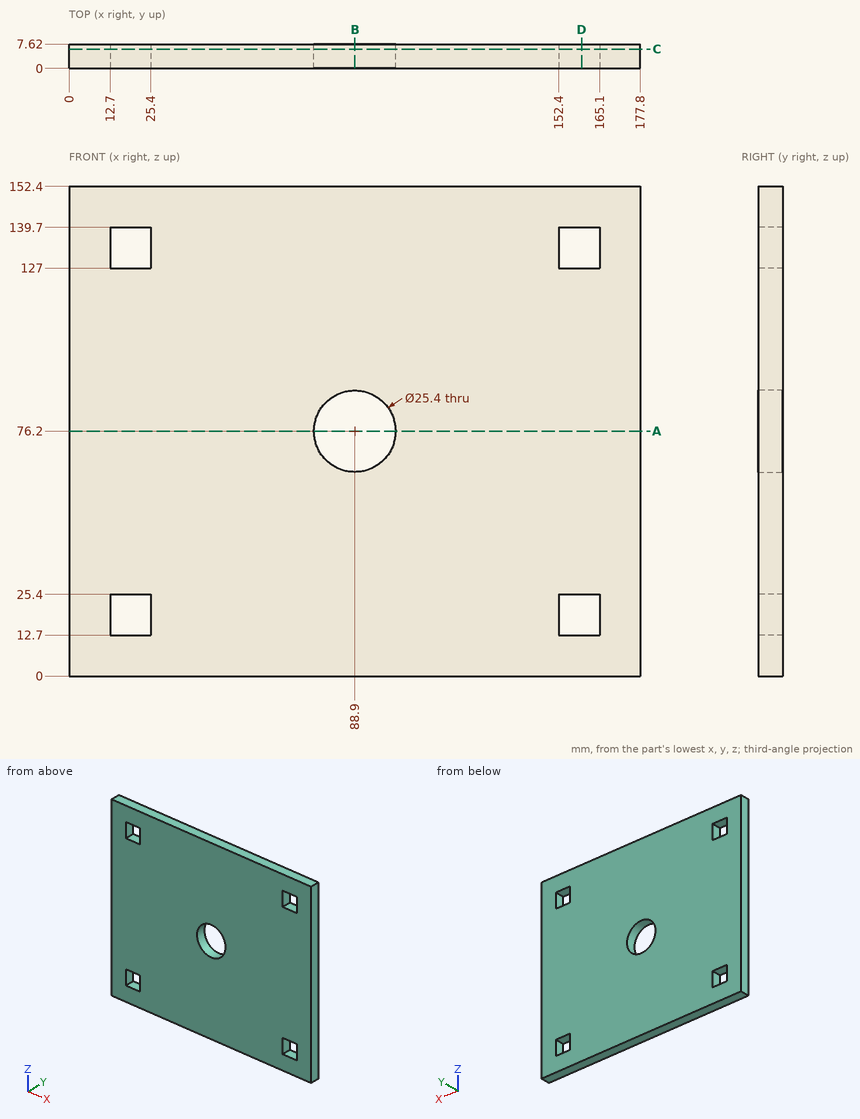
Job drawing, mm, ordinate dimensions from the low corner. One solid piece. Coordinates: 2 decimals unless noted, no trailing zeros. Write each loop counter-clockwise with the first axis right and the second up, starting at its lowest first coordinate (ties: lowest second). Pieces come first, ordered by that corner, then holes.
Item 1: Slice it at D-D (x = 159.5). Write the cut outline in (y, z), and give its area (3 significant figures).
Item 2: Slice it at A-A (z = 76.2). Write the cut outline in (x, y).
Item 3: Slice it at B-B (x = 88.9). Write the cut outline in (y, z).
Item 4: Probe line 1 (X direction, y = 2.5, z = 128.5); line 2 (X direction, y = 4.5, z = 76.2); line 3 (Z direction, x = 80.5, y = 5). List the from-to ranges inside material, lowest first.
Item 5: Slice it at C-C (y = 6). Write the cut outline in (x, z), and give its area (3 significant figures).
Results found:
1. outline: (0, 0) - (7.62, 0) - (7.62, 12.7) - (0, 12.7) - close; (0, 25.4) - (7.62, 25.4) - (7.62, 127) - (0, 127) - close; (0, 139.7) - (7.62, 139.7) - (7.62, 152.4) - (0, 152.4) - close
1. area: 968 mm2
2. outline: (0, 0) - (76.2, 0) - (76.2, 7.62) - (0, 7.62) - close; (101.6, 0) - (177.8, 0) - (177.8, 7.62) - (101.6, 7.62) - close
3. outline: (0, 0) - (7.62, 0) - (7.62, 63.5) - (0, 63.5) - close; (0, 88.9) - (7.62, 88.9) - (7.62, 152.4) - (0, 152.4) - close
4. line 1: x = 0 to 12.7, 25.4 to 152.4, 165.1 to 177.8
4. line 2: x = 0 to 76.2, 101.6 to 177.8
4. line 3: z = 0 to 66.67, 85.73 to 152.4
5. outline: (0, 0) - (177.8, 0) - (177.8, 152.4) - (0, 152.4) - close; hole (12.7, 12.7) - (25.4, 12.7) - (25.4, 25.4) - (12.7, 25.4) - close; hole (12.7, 127) - (25.4, 127) - (25.4, 139.7) - (12.7, 139.7) - close; hole circle Ø25.4 at (88.9, 76.2); hole (152.4, 12.7) - (165.1, 12.7) - (165.1, 25.4) - (152.4, 25.4) - close; hole (152.4, 127) - (165.1, 127) - (165.1, 139.7) - (152.4, 139.7) - close
5. area: 25,900 mm2
